Answer from the drawing. Dimensions are ordinates in mm from the lowest x, y and z of the part. A direction names the side the tool comes from. Coordinates: 2 decimals unless noted, no trailing zeros. Order: outer loops, then holes, each group sorted by start corner. A loop starts at its lowest first (then second) coordinate and runs counter-clockwise, first axis right, second up. Notation, with made-up numbers: (39, -35) - (95, -35) arc R27 cw to (95, -7) - close; hole circle Ø8 at (-17, 88). An arc over 180 degrees is marked (long way). Answer as a JSON object with one key per item and string values. Group by question number.
1) Section B-B (y = 14) is taken. Give the vertices of the cut face in (x, z) (1 decimal), plus the area to 3 significant figures.
2) Section A-A (z = 10.16) is taken. Give the vertices of the cut face in (x, y) (1 decimal).
3) Section D-D (z = 32.5) is taken. Count the separate pieces of the cut face and the enclosed holes in it, plus the area to 3 significant figures.
4) A tool of negligible diameter and unlimited length cuts with its end or side. For the marked faces 1, 2 and 3, from which of +Z, -Z, +X, -X, +Y, -Y can it reach the whole face along a straight path? Write none if from no direction.
5) Section C-C (x = 7.5) is taken. Give the vertices of the cut face in (y, z), plus the area to 3 significant figures.
6) Each of these flat-tipped pins is pushed along its axis until it touches: P1, Ø5.5, axis at y = 3.5, z = 34.5, coming from the +X side; P2, Ø7.5, axis at x = 22.96, y = 22.86, coming from the +Z side; P3, Ø10, axis at x = 20, y = 24.5, coming from the -Z side. Where does it stop, or does it pass through?
7) The mould has two halves that part along X. Classify the marked faces 4, 5, 6 and 7: released by +X, released by -X, zero draft, split by the parting line, or undercut.
8) Find the intervals of material crossed by line 1 along X through (y, z) = (3.6, 10.16) (1 decimal); line 2 along Z through (x, y) = (14.5, 14.5); line 3 along Y through (x, z) = (4.25, 52), in increasing order.
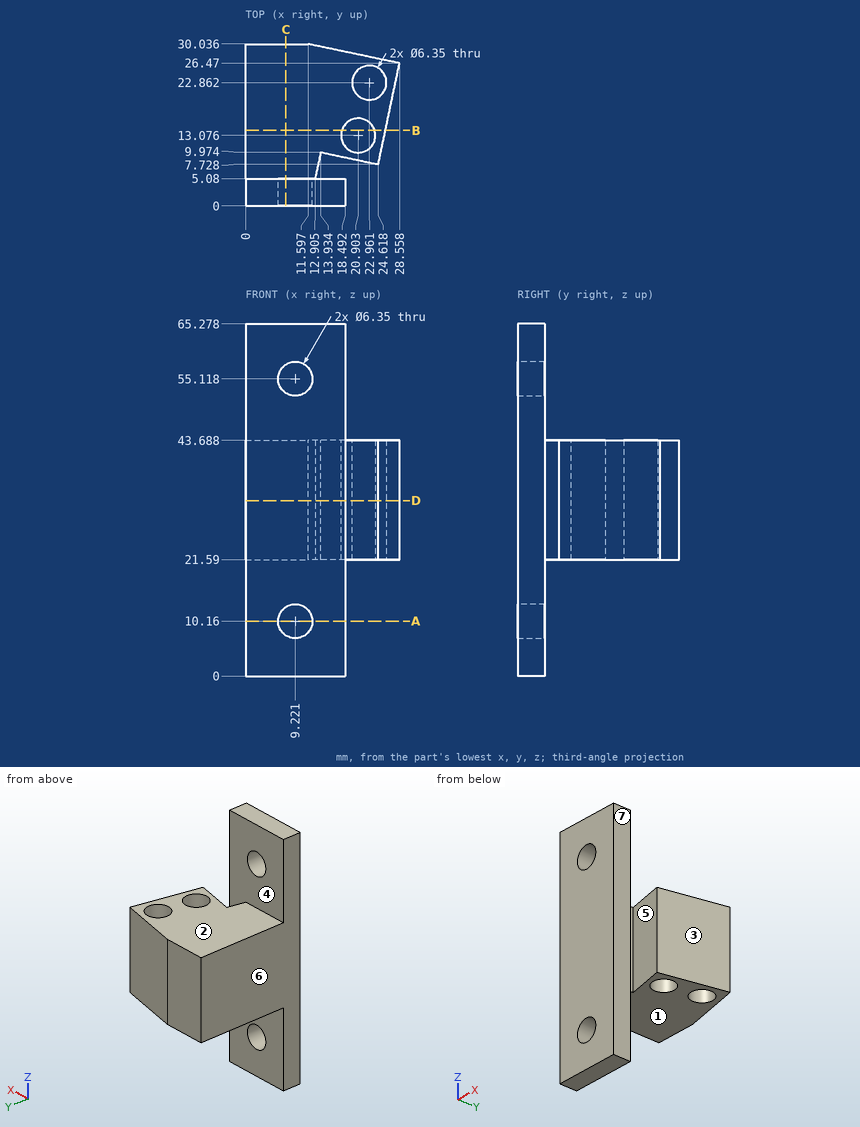
Report:
{
 "1": {"outline": "(0, 21.6) - (17.9, 21.6) - (17.9, 43.7) - (0, 43.7) - close; (23.9, 21.6) - (25.9, 21.6) - (25.9, 43.7) - (23.9, 43.7) - close", "area": "439 mm²"},
 "2": {"outline": "(0, 0) - (6, 0) - (6, 5.1) - (0, 5.1) - close; (12.4, 0) - (18.5, 0) - (18.5, 5.1) - (12.4, 5.1) - close"},
 "3": {"separate pieces": "1", "enclosed holes": "2", "area": "623 mm²"},
 "4": {"face 1": "-Z, +X, -X, +Y", "face 2": "+Z, +X, -X, +Y", "face 3": "+Z, -Z, +X, -Y"},
 "5": {"outline": "(0, 0) - (5.08, 0) - (5.08, 7.49) - (0, 7.49) - close; (0, 12.83) - (5.08, 12.83) - (5.08, 21.59) - (30.04, 21.59) - (30.04, 43.69) - (5.08, 43.69) - (5.08, 52.45) - (0, 52.45) - close; (0, 57.79) - (5.08, 57.79) - (5.08, 65.28) - (0, 65.28) - close", "area": "829 mm²"},
 "6": {"P1": "stops at x = 18.49", "P2": "stops at z = 43.69", "P3": "stops at z = 21.59"},
 "7": {"face 4": "zero draft", "face 5": "undercut", "face 6": "released by -X", "face 7": "released by +X"},
 "8": {"line 1": "x = 0 to 6, 12.4 to 18.5", "line 2": "z = 21.59 to 43.69", "line 3": "y = 0 to 5.08"}
}
